Source: CAD feature listing. Evaluate the final solid. Frame: model axes, mm. Coordinates: 2 decimals unless noted, no trailing zeros. Write each loop counter-clockwise with the first axis right and the second up, starting at its lowest first coordinate (ties: lowest second). Pieces come first, ordered by that corner, then holes. Notation, with made-up numbers: (17, 64) - (54, 64) arc R18 cw to (54, 68) - close; hole circle Ø10 at (53.25, 79.25). An arc over 180 degrees is marked (long way). One line per item, written item: value.
Autodesk Inventor part; units mm, degrees
ref_plane "YZ Plane" through (0, 0, 0) normal (1, 0, 0) x (0, 1, 0)
ref_plane "XZ Plane" through (0, 0, 0) normal (0, 1, 0) x (-1, 0, 0)
ref_plane "XY Plane" through (0, 0, 0) normal (0, 0, 1) x (1, 0, 0)
sketch "Szkic1" plane through (0, 0, 0) normal (0, 0, 1) x (1, 0, 0)
  line L0 (0, 0) -> (6.5, 0)
  line L1 (6.5, 0) -> (6.5, 7.5)
  line L2 (6.5, 7.5) -> (0, 7.5)
  line L3 (0, 7.5) -> (0, 0)
  point P0 (3.25, 4.25)
  dimension "d0" = 6.5
  dimension "d5" = 3.25
  dimension "d6" = 4.25
extrude "Wyciągnięcie proste1" add sketch "Szkic1" along normal mid plane 1
fillet "Zaokrąglenie1" radius 3.25 2 edges at (6.5, 7.5, 0) (0, 7.5, 0)
hole "Otwór1" at (3.25, 4.25, 0) direction (0, 0, -1) diameter 3 end through all both
properties part number "podporka_mala"
1) Contact query for a flat-ended pin moving along its axis: P1, Ø1.5, axis at x = 3.5, y = 4.5, coming from the -Z side. Output: stop coordinate, or through.
Values found:
P1: through
2) Material intervals for line 1 (X direction, y = 4.25, z = 0.1); line 2 (Y direction, x = 3.25, z = -0.2); line 3 (Y direction, x = 4, z = 0.4), sorted ascending.
Values found:
line 1: 0 to 1.75, 4.75 to 6.5
line 2: 0 to 2.75, 5.75 to 7.5
line 3: 0 to 2.95, 5.55 to 7.41
3) Section query A-A on y = 4. Output: boundary loops of the cut face in (x, z), then the cut area to 3 significant figures.
Values found:
outline: (0, -0.5) - (1.77, -0.5) - (1.77, 0.5) - (0, 0.5) - close; (4.73, -0.5) - (6.5, -0.5) - (6.5, 0.5) - (4.73, 0.5) - close
area: 3.54 mm2
4) Draft query along Y for faces 1 (the flat face through (0, 2, 0)), 2 (the cylindrical face through (0.927, 6.523, -0.007)), 3 (the cylindrical face through (1.985, 3.444, -0.007)). Return one class per face: released by +Y, released by -Y, zero draft, split by the parting line, or undercut.
Values found:
face 1: zero draft
face 2: released by +Y
face 3: undercut
5) Section query D-D on y = 6.25. Output: boundary loops of the cut face in (x, z).
Values found:
outline: (0.69, -0.5) - (5.81, -0.5) - (5.81, 0.5) - (0.69, 0.5) - close
6) Section query C-C on x = 2.5. Output: boundary loops of the cut face in (y, z).
Values found:
outline: (0, -0.5) - (2.95, -0.5) - (2.95, 0.5) - (0, 0.5) - close; (5.55, -0.5) - (7.41, -0.5) - (7.41, 0.5) - (5.55, 0.5) - close
